from build123d import *

# Parameters (mm, degrees)
F2_DEPTH = 500


with BuildPart() as f2:
    # F0 (on Front) → F2 (new body)
    with BuildSketch(Plane.XZ):
        with BuildLine():
            Line((0, 50), (0, 0))
            Line((0, 0), (50, 0))
            Line((50, 0), (50, 3))
            ThreePointArc((50, 3), (49.4142135624, 4.4142135624), (48, 5))
            Line((48, 5), (8, 5))
            ThreePointArc((8, 5), (5.8786796564, 5.8786796564), (5, 8))
            Line((5, 8), (5, 48))
            ThreePointArc((5, 48), (4.4142135624, 49.4142135624), (3, 50))
            Line((3, 50), (0, 50))
        make_face()
    extrude(amount=-F2_DEPTH)


solid = f2.part
Here's how the part is built. I have some questions about the finished solid (model axes, mm). A direction names the side the tool comes from. Give positions to 0.01 mm unless a question says otherwise; leave off trailing zeros. Order: outer loops, then holes, each group sorted by start corner. A loop starts at its lowest first (then second) coordinate and runs counter-clockwise, first axis right, second up. Notation, with made-up numbers: (88, 40.25) -> (117, 40.25) arc R15 ccw to (117, 58.25) -> close; hole circle Ø5 at (42.5, -1.75). An arc over 180 degrees is marked (long way). Use a Markdown table: item, result. Add a question column.
Item 1: Imagine slicing it at C-C on x = 33.5. Please give me the cut outline in (y, z), plus the area to 3 significant figures.
Item 2: Imagine slicing it at B-B on z = 15. Please give me the cut outline in (x, y).
Item 3: I need wall thicknesses on line 1 (X direction, y = 52, z = 47); line 2 (Z direction, x = 3.5, y = 318). Which ranges of each line are inside material? Lowest first, please.
Item 4: Will these pins go through, and if not, where does the flat tip stop? pin 1 (6 mm diameter, centred on x = 32.5, y = 404.5, fed in from +Z); pin 2 (5 mm diameter, centred on y = 82, z = 33.5, fed in from +X); pin 3 (8 mm diameter, centred on x = 12.5, z = 24, fed in from +Y).
Item 5: For faces 1 (the face through (28, 246, 5)), 2 (the face through (13.8, 0, 4.7)), which set-ups out of +Z, -Z, +X, -X, +Y, -Y let a thin tool reach every point of the face, with its end or its side?
Item 6: Imagine slicing it at A-A on y = 145.5. Please give me the cut outline in (x, z), plus the area to 3 significant figures.
Data:
| question | item | result |
|---|---|---|
| 1 | outline | (0, 0) -> (500, 0) -> (500, 5) -> (0, 5) -> close |
| 1 | area | 2,500 mm² |
| 2 | outline | (0, 0) -> (5, 0) -> (5, 500) -> (0, 500) -> close |
| 3 | line 1 | x = 0 to 5 |
| 3 | line 2 | z = 0 to 49.94 |
| 4 | pin 1 | stops at z = 5 |
| 4 | pin 2 | stops at x = 5 |
| 4 | pin 3 | passes through |
| 5 | face 1 | +Z, +X, +Y, -Y |
| 5 | face 2 | +Z, -Z, +X, -X, -Y |
| 6 | outline | (0, 0) -> (50, 0) -> (50, 3) arc R2 ccw to (48, 5) -> (8, 5) arc R3 cw to (5, 8) -> (5, 48) arc R2 ccw to (3, 50) -> (0, 50) -> close |
| 6 | area | 475 mm² |
